from build123d import *

# Parameters (mm, degrees)
CROQUIS1_W              = 30
CROQUIS1_H              = 60
CROQUIS1_R              = 3
CROQUIS1_R_2            = 2
CROQUIS1_R_3            = 1.878445215
SALIENTE_EXTRUIR1_DEPTH = 3
CHAFL_N1_SIZE           = 3


with BuildPart() as part:
    # Croquis1 → Saliente-Extruir1 (new body)
    with BuildSketch(Plane(origin=(0, 0, 0), x_dir=(1, 0, 0), z_dir=(0, 1, 0))):
        Rectangle(CROQUIS1_W, CROQUIS1_H)
        with Locations(Location((-10, -17, 0), (0, 0, 270))):
            Circle(CROQUIS1_R, mode=Mode.SUBTRACT)
        with Locations(Location((1, -17, 0), (0, 0, 270))):
            Circle(CROQUIS1_R_2, mode=Mode.SUBTRACT)
        with Locations(Location((10.5, -7.75, 0), (0, 0, 270))):
            Circle(CROQUIS1_R_2, mode=Mode.SUBTRACT)
        with Locations(Location((10.5, -26.25, 0), (0, 0, 270))):
            Circle(CROQUIS1_R_3, mode=Mode.SUBTRACT)
        with BuildLine():
            Line((-10.7, 17.5), (10, 17.5))
            ThreePointArc((10, 17.5), (12.5, 20), (10, 22.5))
            Line((10, 22.5), (-10.7, 22.5))
            ThreePointArc((-10.7, 22.5), (-13.2, 20), (-10.7, 17.5))
        make_face(mode=Mode.SUBTRACT)
    extrude(amount=SALIENTE_EXTRUIR1_DEPTH)

    # Chaflán1
    chafl_n1_edges = [part.edges().sort_by_distance(p)[0] for p in [
        (15, 1.5, 30),
        (-15, 1.5, 30),
        (-15, 1.5, -30),
        (15, 1.5, -30),
    ]]
    chamfer(chafl_n1_edges, length=CHAFL_N1_SIZE)


solid = part.part
Work out the finished part from the listing and answer in its coordinate system (mm). A direction names the side the tool comes from. Give positions to 0.01 mm unless a question says otherwise; leave off trailing zeros. Loops run counter-clockwise (first coordinate to the right, second up) from the corner with the lowest first, then second, coordinate; pieces in that order, holes last. Notation, with made-up numbers: (15.5, 79) - (57.5, 79) arc R21 ccw to (57.5, 95) - close; hole circle Ø10 at (52.25, 70). An arc over 180 degrees is marked (long way). Answer in a Markdown table with one row per item. Add a question column.
Q1. The part is cut by section A-A (z = 17). Determine the outline of the cut face in (x, y).
Q2. A tool of negligible diameter and unlimited length cuts with its end or side. For faces 1 (the flat face through (14, 1, -28)), 2 (the flat face through (0, 1, -17.5)), from which of +Z, -Z, +X, -X, +Y, -Y can it reach the whole face along a straight path? Write none if from no direction.
Q3. Consider line 1 along Z through (x, y) = (6.5, 1.7); line 2 along X through (y, z) = (1.5, 17); line 3 along Z through (x, y) = (-0.75, 0.8). Determine where each line is inside the solid, lowest interval first.
Q4. Determine the mould class of faces 3 (the flat face through (0, 1, -30)), 4 (the flat face through (-13, 1, 29)), 5 (the flat face through (-15, 1, 0)), 6 (the cylindrical face through (10.583, 1.479, 24.373)) for opening direction Z: released by +Z, released by -Z, zero draft, split by the parting line, or undercut.
Q5. The part is cut by section D-D (y = 0.6). Determine the outline of the cut face in (x, z).
Q6. The part is cut by section C-C (z = -20). Determine the outline of the cut face in (x, y).
Q7. The part is cut by section B-B (x = -10). Determine the outline of the cut face in (y, z), and give its area (3 significant figures).
Q8. This flat-tipped pin is pushed along its axis until it touches: P1, Ø3, axis at x = 1, z = 17, coming from the +Y side. Where does it stop, or does it pass through?
Solution:
| question | item | result |
|---|---|---|
| 1 | outline | (-15, 0) - (-13, 0) - (-13, 3) - (-15, 3) - close; (-7, 0) - (-1, 0) - (-1, 3) - (-7, 3) - close; (3, 0) - (15, 0) - (15, 3) - (3, 3) - close |
| 2 | face 1 | -Z, +X, +Y, -Y |
| 2 | face 2 | +Y, -Y |
| 3 | line 1 | z = -30 to -22.5, -17.5 to 30 |
| 3 | line 2 | x = -15 to -13, -7 to -1, 3 to 15 |
| 3 | line 3 | z = -30 to -22.5, -17.5 to 16.03, 17.97 to 30 |
| 4 | face 3 | released by -Z |
| 4 | face 4 | released by +Z |
| 4 | face 5 | zero draft |
| 4 | face 6 | undercut |
| 5 | outline | (-15, -27) - (-12, -30) - (12, -30) - (15, -27) - (15, 27) - (12, 30) - (-12, 30) - (-15, 27) - close; hole circle Ø6 at (-10, 17); hole (-10.7, -22.5) - (10, -22.5) arc R2.5 ccw to (10, -17.5) - (-10.7, -17.5) arc R2.5 ccw to start; hole circle Ø4 at (1, 17); hole circle Ø4 at (10.5, 7.75); hole circle Ø3.76 at (10.5, 26.25) |
| 6 | outline | (-15, 0) - (-13.2, 0) - (-13.2, 3) - (-15, 3) - close; (12.5, 0) - (15, 0) - (15, 3) - (12.5, 3) - close |
| 7 | outline | (0, -30) - (3, -30) - (3, -22.5) - (0, -22.5) - close; (0, -17.5) - (3, -17.5) - (3, 14) - (0, 14) - close; (0, 20) - (3, 20) - (3, 30) - (0, 30) - close |
| 7 | area | 147 mm² |
| 8 | P1 | passes through |
